For this review, use the dimensioned drawing (mm, ordinates from the lowest corner) and the shaded views. A direction names the side the tool comes from. Give positions to 0.01 mm unless a question says otherwise; leave off trailing zeros. Order: outer loops, then holes, each group sorted by start corner. A loop starts at its lowest first (then second) coordinate and runs counter-clockwise, first axis right, second up. Notation, with made-up numbers: M 34.5,-36.75 L 38.5,-36.75 A11 cw 38.5,-23.75 Z; hole C 85,-16.5 d7. An arc over 180 degrees is marked long. Use CSV: the item, a comma, the result in double quotes. Start each with the question number.
(1) Wall thickness on L1, parallel to Z at x = 1.25, y = 20.5; L2, parallel to Y at x = 9, z = 34; L3, parallel to Y at x = 8, z = 32: over which ranges is each line inside the solid? List them lowest first. Write a range as from..to.
(2) Consider section B-B (z = 27.5). Write out the cut boundary in (x, y), and give its area (3 significant figures).
(3) Consider section D-D (z = 37). Write out the cut boundary in (x, y).
(4) Tool access review of the marked faces 1 and 2: name each direction out of +Z, -Z, +X, -X, +Y, -Y from which nothing blocks a thin tool from reaching the whole face with its end or side.
(5) Consider section C-C (y = 18.25). Write out the cut boundary in (x, z), and give its area (3 significant figures).
(6) Clearance check with flat-ended pins moving along their axes: P1, Ø3, axis at y = 21.5, z = 21.5, coming from the -X side (3 decimals); P2, Ø4, axis at x = 2.5, y = 2.5, coming from the +Z side. State where each tip first meets the part, or that it passes through.
(7) Consider section A-A (x = 9.25). Write out the cut boundary in (y, z), and give its area (3 significant figures).
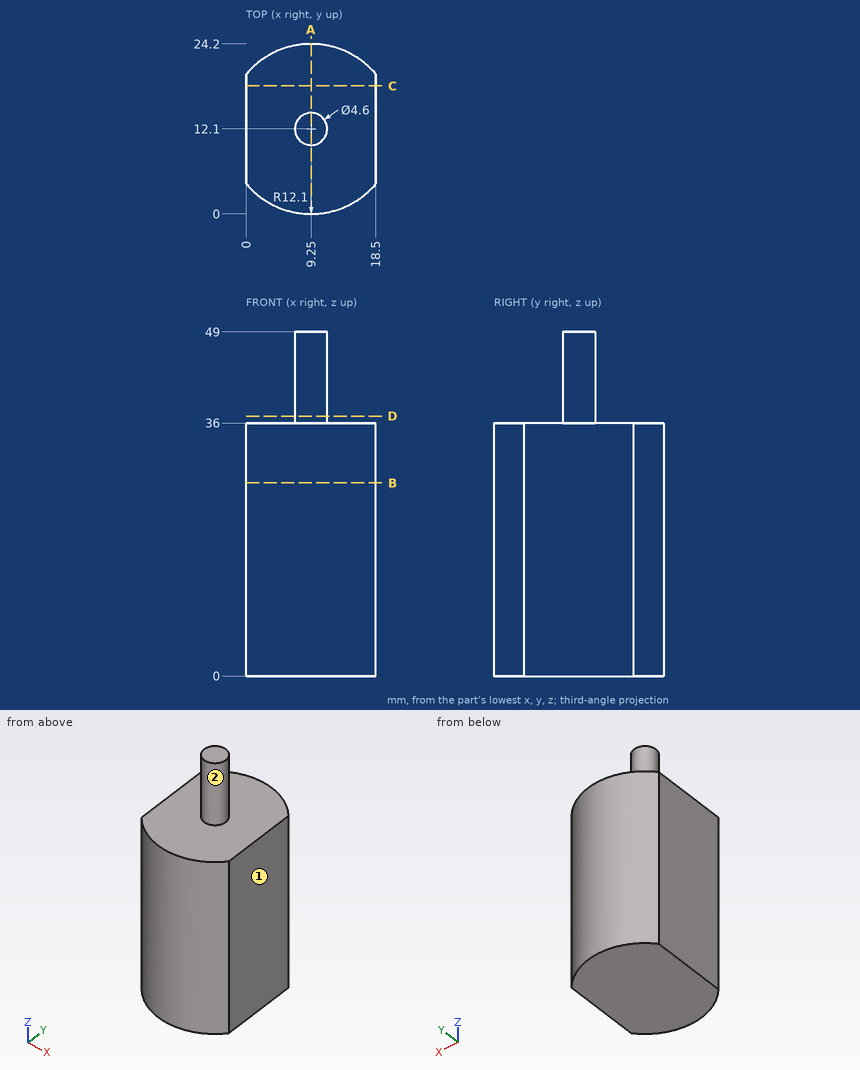
Check result:
1,L1,"z = 0..36"
1,L2,"y = 0..24.2"
1,L3,"y = 0.06..24.14"
2,outline,"M 0,4.3 A12.1 ccw 18.5,4.3 L 18.5,19.9 A12.1 ccw 0,19.9 Z"
2,area,"399 mm^2"
3,outline,"C 9.25,12.1 d4.6"
4,face 1,"+Z, -Z, +X, +Y, -Y"
4,face 2,"+Z"
5,outline,"M 0,0 L 18.5,0 L 18.5,36 L 0,36 Z"
5,area,"666 mm^2"
6,P1,"stops at x = 0.085"
6,P2,"stops at z = 36"
7,outline,"M 0,0 L 24.2,0 L 24.2,36 L 14.4,36 L 14.4,49 L 9.8,49 L 9.8,36 L 0,36 Z"
7,area,"931 mm^2"
